Could you check a few things on this model? Use its own coordinates, in mm. A direction names the side the tool comes from. Give positions to 0.01 mm unless a question says otherwise; leave off trailing zeros. Order: outer loops, then holes, each group sorted by start corner. A loop starts at its lowest first (then second) coordinate and runs counter-clockwise, first axis right, second up.
(1) If I drill on probe 1 along Z at (x, y) = (7.25, 2); probe 2 along X at (y, z) = (-4.5, 3); probe 3 along Z at (x, y) = (1.5, -6), over which ranges is the centre line in solid material (lowest first)?
(2) Imagine slicing it at B-B, the plane z = 3. Write out the boundary of the cut face in (x, y), then the cut area to 3 significant figures.
(3) On a 3-axis mill with a long thin cutter (end or side, diameter ignored), from which of +Z, -Z, +X, -X, +Y, -Y can I reach the whole of each face in a straight line? I mean faces 5 (the cylindrical face through (0.438, 5.483, 9.451)), 6 (the cylindrical face through (5.546, 2.29, 9.451)), 7 (the cylindrical face through (-2.29, 5.546, 9.451)), 8 (the cylindrical face through (-3.141, -5.112, 9.451)), 9 (the cylindrical face through (5.112, -3.141, 9.451)). Say none if no direction works.
(4) Imagine slicing it at A-A, the plane x = -6.25. Write out the boundary of the cut face in (y, z), then the cut area to 3 significant figures.
(5) If we mould it in two halves opening along Y, with no side actions, what happens to faces 1 (the cylindrical face through (-0.65, -4.88, 4.57)), 2 (the cylindrical face through (-5.112, 3.141, 9.451)), 3 (the cylindrical face through (5.35, 1.28, 9.45)), 4 (the cylindrical face through (0.464, -5.982, 9.451))? For each: released by +Y, released by -Y, zero draft, split by the parting line, or undercut.
(6) Will these pins go through, and if not, where does the flat tip stop? pin 1 (3 mm diameter, centred on x = 0, z = 3, fed in from -Y); pin 2 (1 mm diameter, centred on x = -3, z = 10, fed in from -Y); pin 3 (0.6 mm diameter, centred on x = -5.5, z = 8.5, fed in from +Y).
from build123d import *

# Parameters (mm, degrees)
SKETCH1_R           = 8
BOSS_EXTRUDE1_DEPTH = 6
BOSS_EXTRUDE2_DEPTH = 7
SKETCH3_R           = 8
BOSS_EXTRUDE3_DEPTH = 1
SKETCH4_R           = 2.5
CUT_EXTRUDE1_DEPTH  = 19
SKETCH5_R           = 1.7
CUT_EXTRUDE2_DEPTH  = 19


with BuildPart() as part:
    # Sketch1 → Boss-Extrude1 (new body)
    with BuildSketch(Plane.XY):
        Circle(SKETCH1_R)
    extrude(amount=BOSS_EXTRUDE1_DEPTH)

    # Sketch2 → Boss-Extrude2 (add)
    with BuildSketch(Plane.XY.offset(6)):
        with BuildLine():
            Line((0, 5.5), (0, 6))
            ThreePointArc((0, 6), (-0.470754574, 5.981504002), (-0.93860679, 5.926130044))
            Line((-0.93860679, 5.926130044), (-0.860389558, 5.432285873))
            ThreePointArc((-0.860389558, 5.432285873), (-1.283949501, 5.348034562), (-1.699593469, 5.23081084))
            Line((-1.699593469, 5.23081084), (-1.854101966, 5.706339098))
            ThreePointArc((-1.854101966, 5.706339098), (-2.296100594, 5.543277195), (-2.723942998, 5.346039145))
            Line((-2.723942998, 5.346039145), (-2.496947749, 4.900535883))
            ThreePointArc((-2.496947749, 4.900535883), (-2.873742106, 4.689520904), (-3.232818888, 4.449593469))
            Line((-3.232818888, 4.449593469), (-3.526711514, 4.854101966))
            ThreePointArc((-3.526711514, 4.854101966), (-3.89668829, 4.562435794), (-4.242640687, 4.242640687))
            Line((-4.242640687, 4.242640687), (-3.889087297, 3.889087297))
            ThreePointArc((-3.889087297, 3.889087297), (-4.182232811, 3.571964266), (-4.449593469, 3.232818888))
            Line((-4.449593469, 3.232818888), (-4.854101966, 3.526711514))
            ThreePointArc((-4.854101966, 3.526711514), (-5.115840986, 3.134991388), (-5.346039145, 2.723942998))
            Line((-5.346039145, 2.723942998), (-4.900535883, 2.496947749))
            ThreePointArc((-4.900535883, 2.496947749), (-5.081337429, 2.104758878), (-5.23081084, 1.699593469))
            Line((-5.23081084, 1.699593469), (-5.706339098, 1.854101966))
            ThreePointArc((-5.706339098, 1.854101966), (-5.834219522, 1.400672183), (-5.926130044, 0.93860679))
            Line((-5.926130044, 0.93860679), (-5.432285873, 0.860389558))
            ThreePointArc((-5.432285873, 0.860389558), (-5.483045336, 0.431525027), (-5.5, 0))
            Line((-5.5, 0), (-6, 0))
            ThreePointArc((-6, 0), (-5.981504002, -0.470754574), (-5.926130044, -0.93860679))
            Line((-5.926130044, -0.93860679), (-5.432285873, -0.860389558))
            ThreePointArc((-5.432285873, -0.860389558), (-5.348034562, -1.283949501), (-5.23081084, -1.699593469))
            Line((-5.23081084, -1.699593469), (-5.706339098, -1.854101966))
            ThreePointArc((-5.706339098, -1.854101966), (-5.543277195, -2.296100594), (-5.346039145, -2.723942998))
            Line((-5.346039145, -2.723942998), (-4.900535883, -2.496947749))
            ThreePointArc((-4.900535883, -2.496947749), (-4.689520904, -2.873742106), (-4.449593469, -3.232818888))
            Line((-4.449593469, -3.232818888), (-4.854101966, -3.526711514))
            ThreePointArc((-4.854101966, -3.526711514), (-4.562435794, -3.89668829), (-4.242640687, -4.242640687))
            Line((-4.242640687, -4.242640687), (-3.889087297, -3.889087297))
            ThreePointArc((-3.889087297, -3.889087297), (-3.571964266, -4.182232811), (-3.232818888, -4.449593469))
            Line((-3.232818888, -4.449593469), (-3.526711514, -4.854101966))
            ThreePointArc((-3.526711514, -4.854101966), (-3.134991388, -5.115840986), (-2.723942998, -5.346039145))
            Line((-2.723942998, -5.346039145), (-2.496947749, -4.900535883))
            ThreePointArc((-2.496947749, -4.900535883), (-2.104758878, -5.081337429), (-1.699593469, -5.23081084))
            Line((-1.699593469, -5.23081084), (-1.854101966, -5.706339098))
            ThreePointArc((-1.854101966, -5.706339098), (-1.400672183, -5.834219522), (-0.93860679, -5.926130044))
            Line((-0.93860679, -5.926130044), (-0.860389558, -5.432285873))
            ThreePointArc((-0.860389558, -5.432285873), (-0.431525027, -5.483045336), (0, -5.5))
            Line((0, -5.5), (0, -6))
            ThreePointArc((0, -6), (0.470754574, -5.981504002), (0.93860679, -5.926130044))
            Line((0.93860679, -5.926130044), (0.860389558, -5.432285873))
            ThreePointArc((0.860389558, -5.432285873), (1.283949501, -5.348034562), (1.699593469, -5.23081084))
            Line((1.699593469, -5.23081084), (1.854101966, -5.706339098))
            ThreePointArc((1.854101966, -5.706339098), (2.296100594, -5.543277195), (2.723942998, -5.346039145))
            Line((2.723942998, -5.346039145), (2.496947749, -4.900535883))
            ThreePointArc((2.496947749, -4.900535883), (2.873742106, -4.689520904), (3.232818888, -4.449593469))
            Line((3.232818888, -4.449593469), (3.526711514, -4.854101966))
            ThreePointArc((3.526711514, -4.854101966), (3.89668829, -4.562435794), (4.242640687, -4.242640687))
            Line((4.242640687, -4.242640687), (3.889087297, -3.889087297))
            ThreePointArc((3.889087297, -3.889087297), (4.182232811, -3.571964266), (4.449593469, -3.232818888))
            Line((4.449593469, -3.232818888), (4.854101966, -3.526711514))
            ThreePointArc((4.854101966, -3.526711514), (5.115840986, -3.134991388), (5.346039145, -2.723942998))
            Line((5.346039145, -2.723942998), (4.900535883, -2.496947749))
            ThreePointArc((4.900535883, -2.496947749), (5.081337429, -2.104758878), (5.23081084, -1.699593469))
            Line((5.23081084, -1.699593469), (5.706339098, -1.854101966))
            ThreePointArc((5.706339098, -1.854101966), (5.834219522, -1.400672183), (5.926130044, -0.93860679))
            Line((5.926130044, -0.93860679), (5.432285873, -0.860389558))
            ThreePointArc((5.432285873, -0.860389558), (5.483045336, -0.431525027), (5.5, 0))
            Line((5.5, 0), (6, 0))
            ThreePointArc((6, 0), (5.981504002, 0.470754574), (5.926130044, 0.93860679))
            Line((5.926130044, 0.93860679), (5.432285873, 0.860389558))
            ThreePointArc((5.432285873, 0.860389558), (5.348034562, 1.283949501), (5.23081084, 1.699593469))
            Line((5.23081084, 1.699593469), (5.706339098, 1.854101966))
            ThreePointArc((5.706339098, 1.854101966), (5.543277195, 2.296100594), (5.346039145, 2.723942998))
            Line((5.346039145, 2.723942998), (4.900535883, 2.496947749))
            ThreePointArc((4.900535883, 2.496947749), (4.689520904, 2.873742106), (4.449593469, 3.232818888))
            Line((4.449593469, 3.232818888), (4.854101966, 3.526711514))
            ThreePointArc((4.854101966, 3.526711514), (4.562435794, 3.89668829), (4.242640687, 4.242640687))
            Line((4.242640687, 4.242640687), (3.889087297, 3.889087297))
            ThreePointArc((3.889087297, 3.889087297), (3.571964266, 4.182232811), (3.232818888, 4.449593469))
            Line((3.232818888, 4.449593469), (3.526711514, 4.854101966))
            ThreePointArc((3.526711514, 4.854101966), (3.134991388, 5.115840986), (2.723942998, 5.346039145))
            Line((2.723942998, 5.346039145), (2.496947749, 4.900535883))
            ThreePointArc((2.496947749, 4.900535883), (2.104758878, 5.081337429), (1.699593469, 5.23081084))
            Line((1.699593469, 5.23081084), (1.854101966, 5.706339098))
            ThreePointArc((1.854101966, 5.706339098), (1.400672183, 5.834219522), (0.93860679, 5.926130044))
            Line((0.93860679, 5.926130044), (0.860389558, 5.432285873))
            ThreePointArc((0.860389558, 5.432285873), (0.431525027, 5.483045336), (0, 5.5))
        make_face()
    extrude(amount=BOSS_EXTRUDE2_DEPTH)

    # Sketch3 → Boss-Extrude3 (add)
    with BuildSketch(Plane.XY.offset(13)):
        Circle(SKETCH3_R)
    extrude(amount=BOSS_EXTRUDE3_DEPTH)

    # Sketch4 → Cut-Extrude1 (cut, through all)
    with BuildSketch(Plane(origin=(0, 0, 0), x_dir=(-1, 0, 0), z_dir=(0, 0, -1))):
        Circle(SKETCH4_R)
    extrude(amount=-CUT_EXTRUDE1_DEPTH, mode=Mode.SUBTRACT)

    # Sketch5 → Cut-Extrude2 (cut, through all)
    with BuildSketch(Plane(origin=(0, 0, 0), x_dir=(1, 0, 0), z_dir=(0, 1, 0))):
        with Locations(Location((0, -3, 0), (0, 0, 270))):
            Circle(SKETCH5_R)
    extrude(amount=-CUT_EXTRUDE2_DEPTH, mode=Mode.SUBTRACT)


solid = part.part
Answer block:
1. probe 1: z = 0 to 6, 13 to 14
1. probe 2: x = -6.61 to -1.7, 1.7 to 6.61
1. probe 3: z = 0 to 2.2, 3.8 to 6, 13 to 14
2. outline: (-1.7, -7.82) - (-1.7, -1.83) arc R2.5 cw (long way) to (1.7, -1.83) - (1.7, -7.82) arc R8 ccw (long way) to start
2. area: 162 mm2
3. face 5: +Y
3. face 6: +X, +Y
3. face 7: -X, +Y
3. face 8: -X, -Y
3. face 9: +X, -Y
4. outline: (-4.99, 0) - (4.99, 0) - (4.99, 6) - (-4.99, 6) - close; (-4.99, 13) - (4.99, 13) - (4.99, 14) - (-4.99, 14) - close
4. area: 69.9 mm2
5. face 1: zero draft
5. face 2: released by +Y
5. face 3: undercut
5. face 4: released by -Y
6. pin 1: stops at y = 2
6. pin 2: stops at y = -5.35
6. pin 3: stops at y = 2.99
